```python
from build123d import *

# Parameters (mm, degrees)
BOSS_EXTRUDE1_DEPTH = 3.175
SKETCH2_R           = 1.5
SKETCH2_R_2         = 1.500000048
CUT_EXTRUDE1_DEPTH  = 99.065877093


with BuildPart() as part:
    # Sketch1 → Boss-Extrude1 (new body)
    with BuildSketch(Plane(origin=(0, 0, 0), x_dir=(1, 0, 0), z_dir=(0, 1, 0))):
        Polygon((-41.275, 0), (-36.368301991, -11.713851401), (-33.466950324, -10.424361771), (-17.857958519, -45.544593333), (-20.759310186, -46.834082962), (-15.601351667, -58.43948963), (-12.7, -60.325), (-5.08, -60.325), (-5.08, -57.15), (5.08, -57.15), (5.08, -60.325), (12.7, -60.325), (15.601351667, -58.43948963), (20.759310186, -46.834082962), (17.857958519, -45.544593333), (33.466950324, -10.424361771), (36.368301991, -11.713851401), (41.275, 0), (41.275, 25.4), (38.1, 25.4), (38.1, 50.8), (41.275, 50.8), (41.275, 88.9), (28.575, 88.9), (28.575, 85.725), (3.175, 85.725), (-3.175, 85.725), (-28.575, 85.725), (-28.575, 88.9), (-41.275, 88.9), (-41.275, 50.8), (-38.1, 50.8), (-38.1, 25.4), (-41.275, 25.4), align=None)
    extrude(amount=BOSS_EXTRUDE1_DEPTH)

    # Sketch2 → Cut-Extrude1 (cut, through all)
    with BuildSketch(Plane(origin=(0, 0, 0), x_dir=(-1, 0, 0), z_dir=(0, -1, 0))):
        with Locations(Location((39.6875, 69.85, 0), (0, 0, 90))):
            Circle(SKETCH2_R)
        with Locations(Location((-8.89, -58.7375, 0), (0, 0, 270))):
            Circle(SKETCH2_R_2)
        with Locations(Location((39.6875, 12.7, 0), (0, 0, 90))):
            Circle(SKETCH2_R_2)
        with Locations((37.496605417, -5.266403252)):
            Circle(SKETCH2_R_2)
        with Locations(Location((16.729655093, -51.992041481, 0), (0, 0, 90))):
            Circle(SKETCH2_R_2)
        with Locations(Location((8.89, -58.7375, 0), (0, 0, 90))):
            Circle(SKETCH2_R_2)
        with Locations(Location((-16.729655093, -51.992041481, 0), (0, 0, 270))):
            Circle(SKETCH2_R_2)
        with Locations((-37.496605417, -5.266403252)):
            Circle(SKETCH2_R_2)
        with Locations(Location((-39.6875, 12.7, 0), (0, 0, 270))):
            Circle(SKETCH2_R_2)
        with Locations(Location((-39.6875, 69.85, 0), (0, 0, 270))):
            Circle(SKETCH2_R)
    extrude(amount=-CUT_EXTRUDE1_DEPTH, mode=Mode.SUBTRACT)


solid = part.part
```
Source: CAD feature listing. Evaluate the final solid. Frame: model axes, mm. A direction names the side the tool comes from. Give positions to 0.01 mm unless a question says otherwise; leave off trailing zeros. Order: outer loops, then holes, each group sorted by start corner. A loop starts at its lowest first (then second) coordinate and runs counter-clockwise, first axis right, second up.
(1) Contact query for flat-ended pins moving along their axis: P1, Ø2.5, axis at x = -8.89, z = 58.74, coming from the +Y side; P2, Ø1, axis at x = 0.5, y = 1.5, coming from the +Z side; P3, Ø1.6, axis at y = 1, z = 59, coming from the +X side; P4, Ø1, axis at x = -40, y = 2, coming from the +Z side. Output: stop coordinate, or through.
(2) Access query for faces 1 (the face through (-38.1, 2, -38)), 2 (the face through (-5.08, 2, 59)), 3 (the face through (40, 2, -50.8)). Directions: +Z, -Z, +X, -X, +Y, -Y. A direction counts if a zero-diameter tool reaches every point of the face in a straight line with its end or side. Return the directions, or none.
(3) Material intervals for line 1 along X through (y, z) = (1.2, -49); line 2 along Z through (x, y) = (10.5, 1.9) (3 decimals); line 3 along Z through (x, y) = (16, 2.85) (3 decimals), sorted ascending.
(4) Section query B-B (z = -12.7). State how many separate pieces and enclosed holes the cut face has, plus the area to 3 significant figures.
(5) Pull-direction query (Z, two-part tool) for faces 4 (the face through (-40, 2, -50.8)), 5 (the face through (-28.575, 2, -87)), 6 (the face through (-37.544, 1.565, 8.908)); classes: +Z half, -Z half, draft (parallel to the pull), parting line (faces both ways), or undercut.
(6) Section query C-C (z = 18). Return the cut outline in (x, y) (3 decimals).
(7) Section query D-D (x = 31.5). Return the cut outline in (y, z) (3 decimals).
Outcome:
1. P1: passes through
1. P2: stops at z = 57.15
1. P3: stops at x = 15.71
1. P4: stops at z = 4.24
2. face 1: -X, +Y, -Y
2. face 2: +Z, +Y, -Y
2. face 3: +X, +Y, -Y
3. line 1: x = -38.1 to 38.1
3. line 2: z = -85.725 to 60.325
3. line 3: z = -85.725 to 50.681, 53.303 to 57.543
4. separate pieces: 3
4. enclosed holes: 0
4. area: 243 mm2
5. face 4: undercut
5. face 5: draft
5. face 6: +Z half
6. outline: (-30.1, 0) - (30.1, 0) - (30.1, 3.175) - (-30.1, 3.175) - close
7. outline: (0, -88.9) - (3.175, -88.9) - (3.175, 14.85) - (0, 14.85) - close
